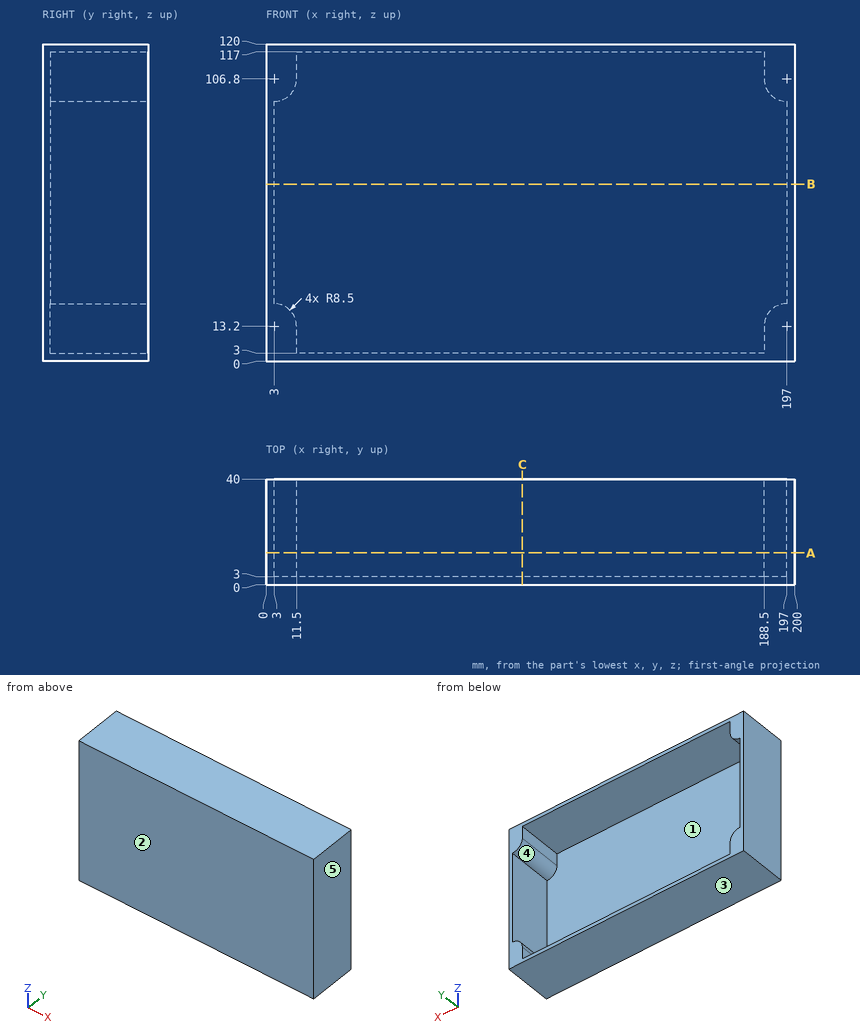
The drawing under review shows one solid part. Ordinate dimensions are in mm from its lowest x, y, z. A direction names the side the tool comes from. Give positions to 0.01 mm unless a question says otherwise; leave off trailing zeros. Write each loop counter-clockwise with the first axis right and the second up, starting at its lowest first coordinate (ties: lowest second). Pieces come first, ordered by that corner, then holes.
1. Tool access review of the marked faces 1 and 2: name each direction out of +Z, -Z, +X, -X, +Y, -Y from which nothing blocks a thin tool from reaching the whole face with its end or side.
2. Add section A-A, the plane y = 12. Write out the cut boundary in (x, z), plus the area to 3 significant figures.
3. Add section C-C, the plane x = 97. Write out the cut boundary in (y, z).
4. Wall thickness on L1, parallel to X at y = 36, z = 88; L2, parallel to Z at x = 20, y = 28; L3, parallel to Y at x = 163.5, z = 33.5: over which ranges is each line inside the solid? List them lowest first.
5. Add section B-B, the plane z = 67. Write out the cut boundary in (x, y).
6. Draft analysis for pull direction Z (two halves, no side actions). For the marked faces 3, 4 and 5, state which applies: +Z half, -Z half, draft (parallel to the pull), parting line (faces both ways), or undercut.
7. For P1, Ø10, axis at x = 131.5, z = 75, coming from the +Y side, flat-tipped, find the tip position at first contact; note if it passes through.
Worked answers:
1. face 1: +Y
1. face 2: +Z, -Z, +X, -X, -Y
2. outline: (0, 0) - (200, 0) - (200, 120) - (0, 120) - close; hole (3, 21.7) arc R8.5 cw to (11.5, 13.2) - (11.5, 3) - (188.5, 3) - (188.5, 13.2) arc R8.5 cw to (197, 21.7) - (197, 98.3) arc R8.5 cw to (188.5, 106.8) - (188.5, 117) - (11.5, 117) - (11.5, 106.8) arc R8.5 cw to (3, 98.3) - close
2. area: 2,460 mm2
3. outline: (0, 0) - (40, 0) - (40, 3) - (3, 3) - (3, 117) - (40, 117) - (40, 120) - (0, 120) - close
4. L1: x = 0 to 3, 197 to 200
4. L2: z = 0 to 3, 117 to 120
4. L3: y = 0 to 3
5. outline: (0, 0) - (200, 0) - (200, 40) - (197, 40) - (197, 3) - (3, 3) - (3, 40) - (0, 40) - close
6. face 3: -Z half
6. face 4: undercut
6. face 5: draft
7. P1: stops at y = 3
